from build123d import *

# Parameters (mm, degrees)
SKETCH1_W           = 100.17
SKETCH1_H           = 80.17
BOSS_EXTRUDE1_DEPTH = 3.175
SKETCH3_R           = 1.415
CUT_EXTRUDE2_DEPTH  = 4.175
SKETCH2_W           = 8.33
SKETCH2_H           = 21.08
CUT_EXTRUDE3_DEPTH  = 10


with BuildPart() as part:
    # Sketch1 → Boss-Extrude1 (new body)
    with BuildSketch(Plane.XY):
        Rectangle(SKETCH1_W, SKETCH1_H)
    extrude(amount=BOSS_EXTRUDE1_DEPTH)

    # Sketch3 → Cut-Extrude2 (cut, through all)
    with BuildSketch(Plane.XY.offset(3.175)):
        with Locations((-44.696699141, 34.696699141)):
            Circle(SKETCH3_R)
        with Locations((44.696699141, 34.696699141)):
            Circle(SKETCH3_R)
        with Locations((44.696699141, -34.696699141)):
            Circle(SKETCH3_R)
        with Locations((-44.696699141, -34.696699141)):
            Circle(SKETCH3_R)
    extrude(amount=-CUT_EXTRUDE2_DEPTH, mode=Mode.SUBTRACT)

    # Sketch2 → Cut-Extrude3 (cut)
    with BuildSketch(Plane.XY.offset(3.175)):
        with Locations((-20.25, 14.675)):
            Rectangle(SKETCH2_W, SKETCH2_H)
        with Locations((20.25, 14.675)):
            Rectangle(SKETCH2_W, SKETCH2_H)
        with Locations((-20.25, -14.675)):
            Rectangle(SKETCH2_W, SKETCH2_H)
        with Locations((20.25, -14.675)):
            Rectangle(SKETCH2_W, SKETCH2_H)
    extrude(amount=-CUT_EXTRUDE3_DEPTH, mode=Mode.SUBTRACT)


solid = part.part
Could you check a few things on this model? Use its own coordinates, in mm. A direction names the side the tool comes from. Round coordinates to 2 decimals unless told otherwise and drop trailing zeros. Order: outer loops, then holes, each group sorted by start corner. A loop starts at its lowest first (then second) coordinate and runs counter-clockwise, first axis right, second up. Notation, with made-up numbers: M 2.5,-12.75 L 31.5,-12.75 A15 cw 31.5,15.25 Z; hole C -12.5,62.25 d8. An arc over 180 degrees is marked long. One line per item, written item: value.
(1) Imagine slicing it at A-A (y = 23). Write out the boundary of the cut face in (x, z) (3 decimals), and give its area (3 significant figures).
Ans:
outline: M -50.085,0 L -24.415,0 L -24.415,3.175 L -50.085,3.175 Z; M -16.085,0 L 16.085,0 L 16.085,3.175 L -16.085,3.175 Z; M 24.415,0 L 50.085,0 L 50.085,3.175 L 24.415,3.175 Z
area: 265 mm^2
(2) Imagine slicing it at B-B (z = 2.65). Count the separate pieces of the cut face and the enclosed holes in it, and give its area (3 significant figures).
Ans:
separate pieces: 1
enclosed holes: 8
area: 7,300 mm^2
(3) I need wall thicknesses on line 1 along X through (y, z) = (-19, 2) (3 decimals); line 2 along Y through (x, z) = (-44.5, 0.8) (3 decimals). Which ranges of each line are inside material? Lowest first, please. Write a range as from..to.
Ans:
line 1: x = -50.085..-24.415, -16.085..16.085, 24.415..50.085
line 2: y = -40.085..-36.098, -33.295..33.295, 36.098..40.085
(4) If we mould it in two halves opening along Y, with no side actions, what happens to faces 1 (the flat face through (-1, 40.085, 2)), 2 (the flat face through (20, -25.215, 2)), 3 (the flat face through (-50.085, -1, 2))? For each: released by +Y, released by -Y, zero draft, split by the parting line, or undercut.
Ans:
face 1: released by +Y
face 2: undercut
face 3: zero draft
(5) Which directions (+Z, -Z, +X, -X, +Y, -Y) give clear straight access to the entire face, cutting with the end or side of a thin tool? Please do faces 4 (the flat face through (-1, 1, 0)), 5 (the flat face through (-24.415, 15, 2)).
Ans:
face 4: -Z, +X, -X, +Y, -Y
face 5: +Z, -Z
(6) I'm going to push a flat-ended pin straight in: P1, Ø1.7, axis at x = 44.7, y = 34.7, coming from the -Z side. Where does the tip first touch, or does it pass through?
Ans:
P1: passes through
